Geometry check sheet. Reference: the model listing, model coordinates, mm. A direction names the side the tool comes from. Give positions to 0.01 mm unless a question says otherwise; leave off trailing zeros. Order: outer loops, then holes, each group sorted by start corner. A loop starts at its lowest first (then second) coordinate and runs counter-clockwise, first axis right, second up. Notation, with made-up numbers: M -16.75,10.25 L -11.75,10.25 A26 cw -11.75,24.25 Z; hole C 85.5,12.25 d2. An arc over 180 degrees is marked long. Answer as CSV lines item,"result".
Autodesk Inventor part; units mm, degrees
ref_plane "YZ Plane" through (0, 0, 0) normal (1, 0, 0) x (0, 1, 0)
ref_plane "XZ Plane" through (0, 0, 0) normal (0, 1, 0) x (-1, 0, 0)
ref_plane "XY Plane" through (0, 0, 0) normal (0, 0, 1) x (1, 0, 0)
sketch "Sketch1" plane through (0, 0, 0) normal (0, 0, 1) x (1, 0, 0)
  line L0 (0, 0) -> (150, 0)
  line L1 (150, 0) -> (150, 80)
  line L2 (150, 80) -> (0, 80)
  line L3 (0, 80) -> (0, 0)
  dimension "d0" = 150
  dimension "d1" = 80
extrude "Extrusion1" add sketch "Sketch1" along normal blind 3
sketch "Sketch2" plane through (0, 0, 3) normal (0, 0, 1) x (1, 0, 0)
  line L0 (0, 80) -> (0, 0)
  line L1 (150, 0) -> (150, 80)
  line L2 (3, 80) -> (3, 53.3333)
  line L3 (3, 53.3333) -> (0, 53.3333)
  line L4 (0, 53.3333) -> (0, 26.6667)
  line L5 (0, 26.6667) -> (3, 26.6667)
  line L6 (3, 26.6667) -> (3, 0)
  line L7 (0, 80) -> (0, 53.3333)
  line L8 (0, 26.6667) -> (0, 0)
  line L9 (147, 80) -> (147, 53.3333)
  line L10 (147, 53.3333) -> (150, 53.3333)
  line L11 (150, 53.3333) -> (150, 26.6667)
  line L12 (150, 26.6667) -> (147, 26.6667)
  line L13 (147, 26.6667) -> (147, 0)
  line L14 (150, 0) -> (150, 26.6667)
  line L15 (150, 53.3333) -> (150, 80)
  line L16 (0, 26.6667) -> (0, 0)
  line L17 (0, 0) -> (0, 3)
  line L18 (0, 3) -> (30, 3)
  line L19 (30, 3) -> (30, 0)
  line L20 (30, 0) -> (60, 0)
  line L21 (0, 0) -> (150, 0)
  line L22 (60, 0) -> (60, 3)
  line L23 (60, 3) -> (90, 3)
  line L24 (90, 3) -> (90, 0)
  line L25 (90, 0) -> (120, 0)
  line L26 (120, 0) -> (120, 3)
  line L27 (120, 3) -> (150, 3)
  line L28 (0, 80) -> (0, 77)
  line L29 (0, 77) -> (30, 77)
  line L30 (30, 77) -> (30, 80)
  line L31 (60, 80) -> (60, 77)
  line L32 (30, 80) -> (60, 80)
  line L33 (0, 80) -> (150, 80)
  line L34 (60, 77) -> (90, 77)
  line L35 (90, 77) -> (90, 80)
  line L36 (120, 80) -> (120, 77)
  line L37 (120, 77) -> (150, 77)
  line L38 (90, 80) -> (120, 80)
  line L39 (0, 0) -> (30, 0)
  line L40 (0, 0) -> (150, 0)
  line L41 (120, 0) -> (150, 0)
  line L42 (150, 0) -> (150, 80)
  line L43 (150, 80) -> (120, 80)
  line L44 (150, 80) -> (0, 80)
  line L45 (30, 80) -> (0, 80)
  dimension "d4" = 3
  dimension "d5" = 26.6667
  dimension "d6" = 26.6667
  dimension "d7" = 3
  dimension "d8" = 26.6667
  dimension "d9" = 26.6667
  dimension "d10" = 3
  dimension "d11" = 30
  dimension "d12" = 30
  dimension "d13" = 30
  dimension "d14" = 30
extrude "Extrusion2" cut sketch "Sketch2" against normal blind 3 contours L33 L2 L29 L0 | L29 L2 L3 L0 | L33 L30 L29 L2 | L5 L6 L18 L0 | L33 L35 L34 L31 | L18 L6 L21 L0 | L18 L19 L21 L6 | L33 L9 L37 L36 | L33 L1 L37 L9 | L37 L1 L10 L9 | L22 L23 L24 L21 | L26 L27 L13 L21 | L1 L27 L13 L12 | L13 L27 L1 L21
sketch "Sketch3" plane through (0, 0, 3) normal (0, 0, 1) x (1, 0, 0)
  line L0 (60, 77) -> (90, 77)
  line L1 (90, 3) -> (60, 3)
  circle A0 centre (75, 40) radius 8.5
  point P0 (0, 0)
  dimension "d17" = 17
extrude "Extrusion3" cut sketch "Sketch3" against normal blind 3
properties part number "TAPA3"
(1) Material ranges on line 1 (X direction, y = 77.5, z = 1.2); line 2 (Y direction, x = 75, z = 1.3); line 3 (Y direction, x = 138.5, z = 1.5), recorded low to high.
The answers:
line 1,"x = 30 to 60, 90 to 120"
line 2,"y = 3 to 31.5, 48.5 to 77"
line 3,"y = 3 to 77"
(2) Draft check along X on faces 1 (the face through (30, 78, 2)), 2 (the face through (133, 77, 2)), 3 (the face through (75, 77, 2)), 4 (the face through (90, 2, 2)). Enter one of: +X half, -X half, draft (parallel to the pull), parting line (faces both ways), or undercut.
The answers:
face 1,"-X half"
face 2,"draft"
face 3,"undercut"
face 4,"undercut"
(3) Tool access check on faces 5 (the face through (16, 77, 2)), 6 (the face through (147, 65, 2)), 7 (the face through (3, 15, 2)). Record the directions out of +Z, -Z, +X, -X, +Y, -Y that give a thin tool (end or side, any length) a straight path to the whole face; none if there is none.
The answers:
face 5,"+Z, -Z, -X, +Y"
face 6,"+Z, -Z, +X, +Y"
face 7,"+Z, -Z, -X, -Y"
(4) Section check D-D on y = 60. Enter the section's corners in (x, z), then the cut area to 3 significant figures.
The answers:
outline,"M 3,0 L 147,0 L 147,3 L 3,3 Z"
area,"432 mm2"
(5) Section check B-B on y = 40. Enter the section's corners in (x, z).
The answers:
outline,"M 0,0 L 66.5,0 L 66.5,3 L 0,3 Z; M 83.5,0 L 150,0 L 150,3 L 83.5,3 Z"
(6) Section check A-A on x = 75. Enter the section's corners in (y, z).
The answers:
outline,"M 3,0 L 31.5,0 L 31.5,3 L 3,3 Z; M 48.5,0 L 77,0 L 77,3 L 48.5,3 Z"
(7) Gauge pin test, flat ends, axial feed: P1, Ø1.5, axis at y = 78, z = 1.5, coming from the -X side; P2, Ø1.5, axis at x = 77, z = 1, coming from the +Y side; P3, Ø0.9, axis at y = 78, z = 1.5, coming from the +X side. Record the tip position at first contact, or that the pin passes through.
The answers:
P1,"stops at x = 30"
P2,"stops at y = 77"
P3,"stops at x = 120"
